Could you check a few things on this drawing? It's one solid part, dimensions in mm from its lowest x, y, z. A direction names the side the tool comes from. Coordinates: 2 decimals unless noted, no trailing zeros. Loops run counter-clockwise (first coordinate to the right, second up) from the corner with the lowest first, then second, coordinate; pieces in that order, holes last. Notation, with made-up numbers: (-30, 39) -> (-2, 39) arc R16 ccw to (-2, 64) -> close; hole circle Ø6 at (15, -3.5). An arc over 180 degrees is marked (long way). One line per question, with ' | ' between items.
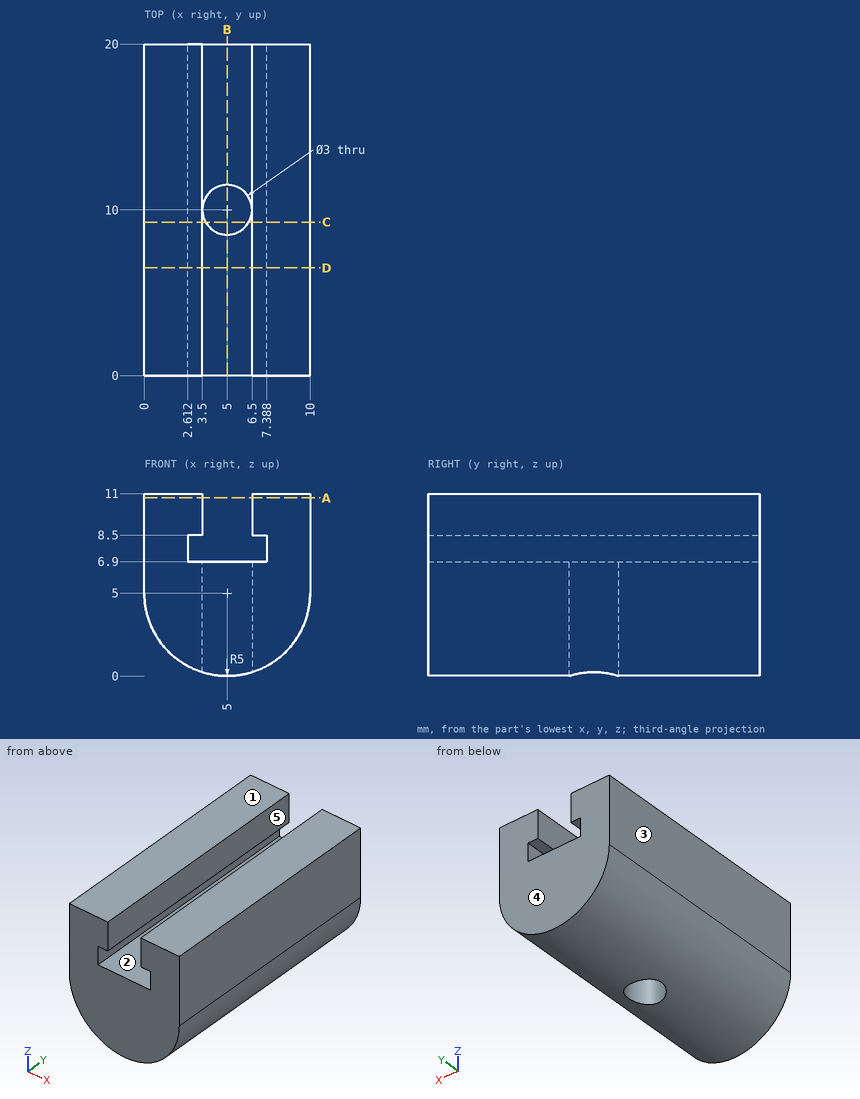
1) I'm going to push a flat-ended pin straight in: pin 1 Ø1 at (x, y) = (3, 13.5) entering from -Z. Where does the tip first touch, or does it pass through?
Data:
pin 1: z = 0.23
2) If we section it at D-D on y = 6.5: Please give me the cut outline in (x, z).
Data:
outline: (0, 5) arc R5 ccw to (10, 5) -> (10, 11) -> (6.5, 11) -> (6.5, 8.5) -> (7.39, 8.5) -> (7.39, 6.9) -> (2.61, 6.9) -> (2.61, 8.5) -> (3.5, 8.5) -> (3.5, 11) -> (0, 11) -> close
3) If we section it at C-C on y = 9.25: Please give me the cut outline in (x, z).
Data:
outline: (0, 5) arc R5 ccw to (3.7, 0.17) -> (3.7, 6.9) -> (2.61, 6.9) -> (2.61, 8.5) -> (3.5, 8.5) -> (3.5, 11) -> (0, 11) -> close; (6.3, 0.17) arc R5 ccw to (10, 5) -> (10, 11) -> (6.5, 11) -> (6.5, 8.5) -> (7.39, 8.5) -> (7.39, 6.9) -> (6.3, 6.9) -> close
4) If we section it at B-B on x = 5: Please give me the cut outline in (y, z).
Data:
outline: (0, 0) -> (8.5, 0) -> (8.5, 6.9) -> (0, 6.9) -> close; (11.5, 0) -> (20, 0) -> (20, 6.9) -> (11.5, 6.9) -> close
5) We'd pull the mould along Z, two halves only. Please class the marked faces 1, 2 and 3: pulls with the +Z half, pulls with the -Z half, needs draft (parallel to the pull), parting line crosses it, or undercut.
Data:
face 1: pulls with the +Z half | face 2: undercut | face 3: needs draft
6) If we section it at A-A on z = 10.75: Please give me the cut outline in (x, y), and give its area (3 significant figures).
Data:
outline: (0, 0) -> (3.5, 0) -> (3.5, 20) -> (0, 20) -> close; (6.5, 0) -> (10, 0) -> (10, 20) -> (6.5, 20) -> close | area: 140 mm²
7) I need wall thicknesses on line 1 along Y through (x, z) = (5, 2.75); line 2 along X through (y, z) = (9, 8.25); line 3 along X through (y, z) = (14, 9). Which ranges of each line are inside material? Lowest first, please. Write a range as from..to.
Data:
line 1: 0..8.5, 11.5..20 | line 2: 0..2.61, 7.39..10 | line 3: 0..3.5, 6.5..10
8) On a 3-axis mill with a long thin cutter (end or side, diameter ignored), from which of +Z, -Z, +X, -X, +Y, -Y can I reach the whole of each face in a straight line? I mean the marked faces 4 and 5. Say none if no direction works.
Data:
face 4: +Z, -Z, +X, -X, +Y | face 5: +Z, +Y, -Y
